```python
from build123d import *

# Parameters (mm, degrees)
CROQUIS1_W                = 71.796950719
CROQUIS1_H                = 66.705557785
SALIENTE_EXTRUIR1_DEPTH   = 10
CORTAR_EXTRUIR1_DEPTH     = 3
CROQUIS4_R                = 2
CORTAR_EXTRUIR3_DEPTH     = 4
CORTAR_EXTRUIR4_START     = -1
CORTAR_EXTRUIR4_OUTLINE_W = 71.796950719
CORTAR_EXTRUIR4_OUTLINE_H = 66.705557785
CORTAR_EXTRUIR4_DEPTH     = 1
CROQUIS6_W                = 10.482335709
CROQUIS6_H                = 10
CORTAR_EXTRUIR5_DEPTH     = 5.2
CROQUIS7_R                = 2
CORTAR_EXTRUIR6_DEPTH     = 6.2
CROQUIS8_W                = 6.4
CROQUIS8_H                = 36.352778893
CORTAR_EXTRUIR7_DEPTH     = 1


# Read off the part's stored shape, not the designer's step: Cortar-Extruir4
with BuildPart() as part:
    # Croquis1 → Saliente-Extruir1 (new body)
    with BuildSketch(Plane(origin=(0, 0, 0), x_dir=(1, 0, 0), z_dir=(0, 1, 0))):
        with Locations((42.262259736, 150.287845226)):
            Rectangle(CROQUIS1_W, CROQUIS1_H)
    extrude(amount=SALIENTE_EXTRUIR1_DEPTH)

    # Croquis3 → Cortar-Extruir1 (cut)
    with BuildSketch(Plane(origin=(0, 10, 0), x_dir=(1, 0, 0), z_dir=(0, 1, 0))):
        with BuildLine():
            Line((33.262259735, 150.310457053), (51.262259735, 150.310457053))
            ThreePointArc((51.262259735, 150.310457053), (56.284871563, 145.287845226), (51.262259735, 140.265233398))
            Line((51.262259735, 140.265233398), (33.262259735, 140.265233398))
            ThreePointArc((33.262259735, 140.265233398), (28.239647907, 145.287845226), (33.262259735, 150.310457053))
        make_face()
    extrude(amount=-CORTAR_EXTRUIR1_DEPTH, mode=Mode.SUBTRACT)

    # Croquis4 → Cortar-Extruir3 (cut)
    with BuildSketch(Plane(origin=(0, 10, 0), x_dir=(1, 0, 0), z_dir=(0, 1, 0))):
        with Locations(Location((51.262259735, 145.287845226, 0), (0, 0, 270))):
            Circle(CROQUIS4_R)
        with Locations(Location((33.262259735, 145.287845226, 0), (0, 0, 270))):
            Circle(CROQUIS4_R)
    extrude(amount=-CORTAR_EXTRUIR3_DEPTH, mode=Mode.SUBTRACT)

    # Cortar-Extruir4 outline → Cortar-Extruir4 (cut)
    with BuildSketch(Plane(origin=(0, 10, 0), x_dir=(1, 0, 0), z_dir=(0, 1, 0)).offset(CORTAR_EXTRUIR4_START)):
        with Locations((42.262259736, 150.287845226)):
            Rectangle(CORTAR_EXTRUIR4_OUTLINE_W, CORTAR_EXTRUIR4_OUTLINE_H)
        with BuildLine():
            ThreePointArc((33.262259735, 140.265233398), (28.239647907, 145.287845226), (33.262259735, 150.310457053))
            Line((33.262259735, 150.310457053), (51.262259735, 150.310457053))
            ThreePointArc((51.262259735, 150.310457053), (56.284871563, 145.287845226), (51.262259735, 140.265233398))
            Line((51.262259735, 140.265233398), (33.262259735, 140.265233398))
        make_face(mode=Mode.SUBTRACT)
    extrude(amount=CORTAR_EXTRUIR4_DEPTH, mode=Mode.SUBTRACT)

    # Croquis6 → Cortar-Extruir5 (cut)
    with BuildSketch(Plane(origin=(0, 10, 0), x_dir=(1, 0, 0), z_dir=(0, 1, 0))):
        with Locations((42.262259736, 145.287845226)):
            Rectangle(CROQUIS6_W, CROQUIS6_H)
    extrude(amount=-CORTAR_EXTRUIR5_DEPTH, mode=Mode.SUBTRACT)

    # Croquis7 → Cortar-Extruir6 (cut)
    with BuildSketch(Plane(origin=(0, 10, 0), x_dir=(1, 0, 0), z_dir=(0, 1, 0))):
        with Locations(Location((42.262259735, 145.287845226, 0), (0, 0, 270))):
            Circle(CROQUIS7_R)
    extrude(amount=-CORTAR_EXTRUIR6_DEPTH, mode=Mode.SUBTRACT)

    # Croquis8 → Cortar-Extruir7 (cut)
    with BuildSketch(Plane(origin=(0, 9, 0), x_dir=(1, 0, 0), z_dir=(0, 1, 0))):
        with Locations((42.262259735, 135.11145578)):
            Rectangle(CROQUIS8_W, CROQUIS8_H)
    extrude(amount=-CORTAR_EXTRUIR7_DEPTH, mode=Mode.SUBTRACT)


solid = part.part
```
Check sheet for the modelled part. Datum: model origin and axes. Units: mm. A direction names the side the tool comes from. Give positions to 0.01 mm unless a question says otherwise; leave off trailing zeros. Answer in a Markdown table with one row per item. Add a question column.
Q1. Thickness scan on L1, parallel to Z at x = 39, y = 6.75; L2, parallel to X at y = 6.75, z = -144.5; L3, parallel to Y at x = 44, z = -126. Record the ranges inside material, lowest first.
Q2. Access from +Z, -Z, +X, -X, +Y, -Y to the whole of each face (thin tool, end or side, straight path). Record for faces 1 (the flat face through (42, 3.8, -145)), 2 (the flat face through (42, 9, -158)).
Q3. Release check for a two-part mould opening along Z. For faces 3 (the flat face through (42, 4, -183.641)), 4 (the flat face through (42, 8, -152)), 5 (the flat face through (33, 6, -145)) record: released by +Z, released by -Z, zero draft, split by the parting line, or undercut.
Q4. Gauge pin test, flat ends, axial feed: pin 1 Ø3 at (x, z) = (41.5, -146.5) entering from +Y; pin 2 Ø5 at (x, z) = (51, -155) entering from -Y; pin 3 Ø4.5 at (x, z) = (34, -146) entering from +Y; pin 4 Ø1.5 at (x, z) = (41.5, -152) entering from +Y. Record the tip position at first contact, or that the pin passes through.
Verdict:
| question | item | result |
|---|---|---|
| 1 | L1 | -183.64 to -150.29, -140.29 to -116.94 |
| 1 | L2 | 6.36 to 31.42, 35.1 to 37.02, 47.5 to 49.42, 53.1 to 78.16 |
| 1 | L3 | 0 to 8 |
| 2 | face 1 | +Y |
| 2 | face 2 | +Z, -Z, +X, -X, +Y |
| 3 | face 3 | released by -Z |
| 3 | face 4 | zero draft |
| 3 | face 5 | undercut |
| 4 | pin 1 | y = 4.8 |
| 4 | pin 2 | y = 0 |
| 4 | pin 3 | y = 7 |
| 4 | pin 4 | y = 8 |
